Can you work these out from the model? Positions are in its coordinate system, mm. Round coordinates to 2 decimals unless told otherwise and drop trailing zeros. Write each loop counter-clockwise with the first axis right and the second up, starting at its lowest first coordinate (ties: lowest second). Pieces come first, ordered by that corner, then holes. Notation, with made-up numbers: M 17.5,-1 L 58.5,-1 A32 cw 58.5,28 Z; hole C -9,-36.75 d10. An arc over 180 degrees is marked long. Answer as a JSON object with one key per item and string values. Group by question number.
1) Suppose I cut it at B-B, the plane x = 75. Write out the boundary of the cut face in (y, z), and give its area (3 significant figures).
2) Suppose I cut it at A-A, the plane y = 203.5. Write out the boundary of the cut face in (x, z).
3) I'm going to push flat-ended pins straight in: pin 1 Ø2 at (y, z) = (301, -11) entering from -X; pin 2 Ø10.5 at (x, y) = (-120, 55) entering from -Z (1 decimal); pin 3 Ø5 at (x, z) = (-10, -10.5) entering from +Y; pin 4 Ø3 at (x, z) = (89.5, 5) entering from +Y. Where does each tip first touch, or does it pass through?
4) Suppose I cut it at D-D, the plane x = 120. Write out the boundary of the cut face in (y, z), and give its area (4 significant figures).
5) Please list where these lines run through material, in increasing order: L1, parallel to X at y = 332, z = 0; L2, parallel to X at y = 251.5, z = 6.5; L3, parallel to X at y = 52, z = -10.5. Write a range as [from, to].
6) Suppose I cut it at C-C, the plane y = 55. Write out the boundary of the cut face in (x, z).
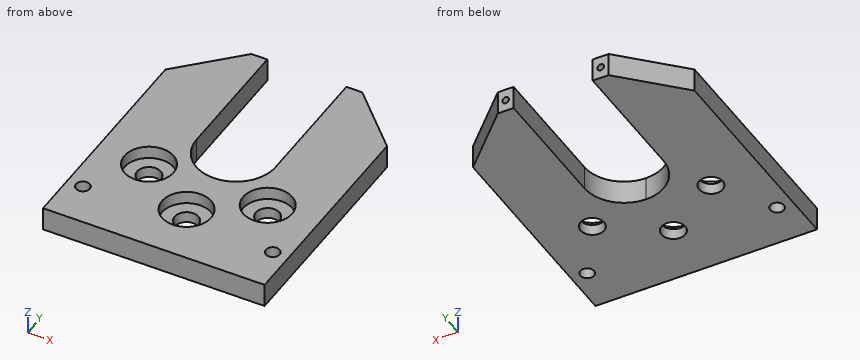
from build123d import *

# Parameters (mm, degrees)
SKETCH2_W              = 280
SKETCH2_H              = 30
BOSS_EXTRUDE2_DEPTH    = 350
CUT_EXTRUDE1_DEPTH     = 350
CHAMFER1_SIZE          = 70
M10_TAPPED_HOLE1_D     = 8.5
M10_TAPPED_HOLE1_DEPTH = 24
M10_TAPPED_HOLE1_TIP   = 4.25
SKETCH8_R              = 8.75
CUT_EXTRUDE2_DEPTH     = 350
SKETCH9_R              = 15
CUT_EXTRUDE3_DEPTH     = 350
SKETCH10_R             = 31
CUT_EXTRUDE4_DEPTH     = 16


with BuildPart() as part:
    # Sketch2 → Boss-Extrude2 (new body)
    with BuildSketch(Plane(origin=(0, 0, 0), x_dir=(1, 0, 0), z_dir=(0, 1, 0))):
        Rectangle(SKETCH2_W, SKETCH2_H)
    extrude(amount=BOSS_EXTRUDE2_DEPTH)

    # Sketch4 → Cut-Extrude1 (cut)
    with BuildSketch(Plane.XY.offset(15)):
        with BuildLine():
            Line((50, 350), (0, 350))
            Line((0, 350), (0, 138))
            ThreePointArc((0, 138), (35.355339059, 152.644660941), (50, 188))
            Line((50, 188), (50, 350))
        make_face()
        with BuildLine():
            Line((0, 138), (0, 350))
            Line((0, 350), (-50, 350))
            Line((-50, 350), (-50, 188))
            ThreePointArc((-50, 188), (-35.355339059, 152.644660941), (0, 138))
        make_face()
        with BuildLine():
            ThreePointArc((50, 350), (35.355339059, 385.355339059), (0, 400))
            Line((0, 400), (0, 350))
            Line((0, 350), (50, 350))
        make_face()
        with BuildLine():
            Line((0, 350), (0, 400))
            ThreePointArc((0, 400), (-35.355339059, 385.355339059), (-50, 350))
            Line((-50, 350), (0, 350))
        make_face()
    extrude(amount=-CUT_EXTRUDE1_DEPTH, mode=Mode.SUBTRACT)

    # Chamfer1
    chamfer1_edges = [part.edges().sort_by_distance(p)[0] for p in [
        (140, 350, 0),
        (-140, 350, 0),
    ]]
    chamfer(chamfer1_edges, length=CHAMFER1_SIZE)

    # M10 Tapped Hole1
    with Locations(Plane(origin=(-60, 350, 0), x_dir=(0, 0, 1), z_dir=(0, 1, 0))):
        with Locations((0, 0), (0, 120)):
            Hole(M10_TAPPED_HOLE1_D / 2, depth=M10_TAPPED_HOLE1_DEPTH)
            with Locations((0, 0, -(M10_TAPPED_HOLE1_DEPTH + M10_TAPPED_HOLE1_TIP / 2))):  # 90° drill point
                Cone(0, M10_TAPPED_HOLE1_D / 2, M10_TAPPED_HOLE1_TIP, mode=Mode.SUBTRACT)

    # Sketch8 → Cut-Extrude2 (cut)
    with BuildSketch(Plane.XY.offset(15)):
        with Locations((-120, 55)):
            Circle(SKETCH8_R)
        with Locations((120, 55)):
            Circle(SKETCH8_R)
    extrude(amount=-CUT_EXTRUDE2_DEPTH, mode=Mode.SUBTRACT)

    # Sketch9 → Cut-Extrude3 (cut)
    with BuildSketch(Plane.XY.offset(15)):
        with Locations((-75, 124.749371855)):
            Circle(SKETCH9_R)
        with Locations((75, 124.749371855)):
            Circle(SKETCH9_R)
        with Locations((0, 75)):
            Circle(SKETCH9_R)
    extrude(amount=-CUT_EXTRUDE3_DEPTH, mode=Mode.SUBTRACT)

    # Sketch10 → Cut-Extrude4 (cut)
    with BuildSketch(Plane.XY.offset(15)):
        with Locations((-75, 124.749371855)):
            Circle(SKETCH10_R)
        with Locations((0, 75)):
            Circle(SKETCH10_R)
        with Locations((75, 124.749371855)):
            Circle(SKETCH10_R)
    extrude(amount=-CUT_EXTRUDE4_DEPTH, mode=Mode.SUBTRACT)


solid = part.part
Results:
{
 "1": {"outline": "M 0,-15 L 109.75,-15 L 109.75,-1 L 93.75,-1 L 93.75,15 L 0,15 Z; M 139.75,-15 L 345,-15 L 345,15 L 155.75,15 L 155.75,-1 L 139.75,-1 Z", "area": "8,940 mm^2"},
 "2": {"outline": "M -140,-15 L -50,-15 L -50,15 L -140,15 Z; M 50,-15 L 140,-15 L 140,15 L 50,15 Z"},
 "3": {"pin 1": "x = -120", "pin 2": "through", "pin 3": "y = 139.59", "pin 4": "y = 332"},
 "4": {"outline": "M 0,-15 L 46.25,-15 L 46.25,15 L 0,15 Z; M 63.75,-15 L 300,-15 L 300,15 L 63.75,15 Z", "area": "8,475 mm^2"},
 "5": {"L1": "[-88, -64.25], [-55.75, -50], [50, 55.75], [64.25, 88]", "L2": "[-140, -50], [50, 140]", "L3": "[-140, -128.22], [-111.78, 111.78], [128.22, 140]"},
 "6": {"outline": "M -140,-15 L -128.75,-15 L -128.75,15 L -140,15 Z; M -111.25,-15 L 111.25,-15 L 111.25,15 L 23.69,15 L 23.69,-1 L -23.69,-1 L -23.69,15 L -111.25,15 Z; M 128.75,-15 L 140,-15 L 140,15 L 128.75,15 Z"}
}
